Geometry: final body of the model. Coordinates: model frame, mm. Face numbers are marked on the shaded views. A direction names the side the tool comes from. Coordinates: 2 decimals unless noted, no trailing zeros. Write each loop counter-clockwise with the first axis right and the second up, starting at its lowest first coordinate (ties: lowest second). Pieces come first, ordered by that corner, then holes. Notation, with made-up numbers: (40.25, 46.25) -> (47.25, 46.25) arc R28 ccw to (47.25, 70.25) -> close; hole circle Ø8 at (38.5, -2). An arc over 180 degrees is marked (long way). One line per item, written item: value.
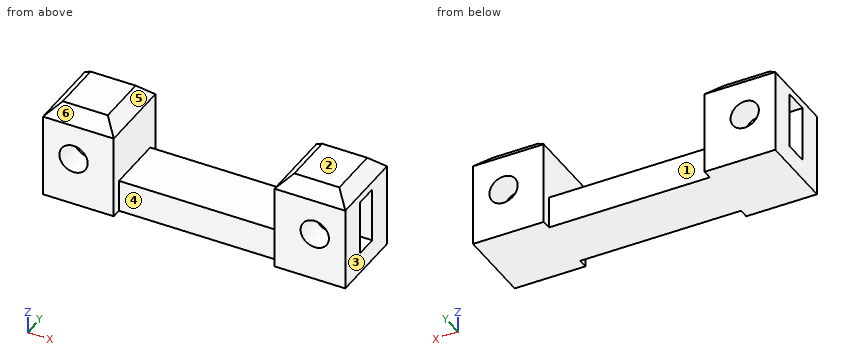
```python
from build123d import *

# Parameters (mm, degrees)
F0_R     = 2.2
F1_DEPTH = 12
F2_W     = 3.5
F2_H     = 8.5
F3_DEPTH = 9.5
F4_W     = 3.7
F4_H     = 8.7
F5_DEPTH = 9.5
F6_W     = 25
F6_H     = 1.5
F7_DEPTH = 5.001
F8_SIZE  = 2


with BuildPart() as f1:
    # F0 (on Front) → F1 (new body)
    with BuildSketch(Plane.XZ):
        Polygon((11, 15), (0, 15), (0, 0), (47, 0), (47, 15), (36, 15), (36, 5), (11, 5), align=None)
        with Locations((4.75, 7.5)):
            Circle(F0_R, mode=Mode.SUBTRACT)
        with Locations((42.25, 7.5)):
            Circle(F0_R, mode=Mode.SUBTRACT)
    extrude(amount=F1_DEPTH)

    # F2 (on face) → F3 (cut)
    with BuildSketch(Plane.YZ.offset(47)):
        with Locations((-6, 7.5)):
            Rectangle(F2_W, F2_H)
    extrude(amount=-F3_DEPTH, mode=Mode.SUBTRACT)

    # F4 (on face) → F5 (cut)
    with BuildSketch(Plane(origin=(0, 0, 0), x_dir=(0, -1, 0), z_dir=(-1, 0, 0))):
        with Locations((6, 7.5)):
            Rectangle(F4_W, F4_H)
    extrude(amount=-F5_DEPTH, mode=Mode.SUBTRACT)

    # F6 (on face) → F7 (cut, through all)
    with BuildSketch(Plane.XY.offset(5)):
        with Locations((23.5, -0.75)):
            Rectangle(F6_W, F6_H)
        with Locations((23.5, -11.25)):
            Rectangle(F6_W, F6_H)
    extrude(amount=-F7_DEPTH, mode=Mode.SUBTRACT)

    # F8
    f8_edges = [f1.edges().sort_by_distance(p)[0] for p in [
        (11, -6, 15),
        (0, -6, 15),
        (5.5, 0, 15),
        (5.5, -12, 15),
        (47, -6, 15),
        (36, -6, 15),
        (41.5, 0, 15),
        (41.5, -12, 15),
    ]]
    chamfer(f8_edges, length=F8_SIZE)


solid = f1.part
```
(1) Section B-B (z = 7.5). State how many separate pieces and enclosed holes the cut face has, then the cut area to 3 significant figures.
Responses:
separate pieces: 6
enclosed holes: 0
area: 122 mm2
(2) Section A-A (x = 42.25). Return the cut outline in (y, z), then the cut area to 3 significant figures.
Responses:
outline: (-12, 0) -> (0, 0) -> (0, 5.3) -> (-4.25, 5.3) -> (-4.25, 3.25) -> (-7.75, 3.25) -> (-7.75, 5.3) -> (-12, 5.3) -> close; (-12, 9.7) -> (-7.75, 9.7) -> (-7.75, 11.75) -> (-4.25, 11.75) -> (-4.25, 9.7) -> (0, 9.7) -> (0, 13) -> (-2, 15) -> (-10, 15) -> (-12, 13) -> close
area: 109 mm2
(3) Pull-direction query (X, two-part tool) for the marked faces 1, 2 and 3; classes: released by +X, released by -X, zero draft, split by the parting line, or undercut.
Responses:
face 1: undercut
face 2: zero draft
face 3: released by +X
(4) Line query: line 1 (X direction, y = -1.25, z = 7.5); line 2 (X direction, y = -1.25, z = 12); line 3 (X direction, y = -11.5, z = 9). Output: solid intervals per line, ascending. Write a range as [from, to].
Responses:
line 1: x = [0, 2.55], [6.95, 11], [36, 40.05], [44.45, 47]
line 2: x = [0, 11], [36, 47]
line 3: x = [0, 3.14], [6.36, 11], [36, 40.64], [43.86, 47]
(5) Section D-D (x = 4.75). Return the cut outline in (y, z).
Responses:
outline: (-12, 0) -> (0, 0) -> (0, 5.3) -> (-4.15, 5.3) -> (-4.15, 3.15) -> (-7.85, 3.15) -> (-7.85, 5.3) -> (-12, 5.3) -> close; (-12, 9.7) -> (-7.85, 9.7) -> (-7.85, 11.85) -> (-4.15, 11.85) -> (-4.15, 9.7) -> (0, 9.7) -> (0, 13) -> (-2, 15) -> (-10, 15) -> (-12, 13) -> close
(6) First-contact query: pin 1 (4.5 mm diameter, centred on x = 19, y = -6, fed in from +Z); pin 2 (2 mm diameter, centred on y = -5.5, z = 7.5, fed in from +X); pin 3 (1.1 mm diameter, centred on y = -6.5, z = 8.5, fed in from -X). Flat tips, straight axial feed; report the tip coordinate or a pass-through.
Responses:
pin 1: stops at z = 5
pin 2: stops at x = 37.5
pin 3: stops at x = 9.5
(7) Section C-C (y = -4.75). Return the cut outline in (x, z), then the cut area to 3 significant figures.
Responses:
outline: (0, 0) -> (47, 0) -> (47, 3.25) -> (37.5, 3.25) -> (37.5, 11.75) -> (47, 11.75) -> (47, 13) -> (45, 15) -> (38, 15) -> (36, 13) -> (36, 5) -> (11, 5) -> (11, 13) -> (9, 15) -> (2, 15) -> (0, 13) -> (0, 11.85) -> (9.5, 11.85) -> (9.5, 3.15) -> (0, 3.15) -> close
area: 284 mm2
(8) Reachability of the marked faces 4, 5 and 6 from +Z, -Z, +X, -X, +Y, -Y: full face, straight path, thin tool, end or side. Return the list, or none.
Responses:
face 4: +Z, -Z, -Y
face 5: +Z, +Y, -Y
face 6: +Z, +X, -X, -Y
